Check sheet for the modelled part. Datum: model origin and axes. Units: mm. A direction names the side the tool comes from. Coordinates: 2 decimals unless noted, no trailing zeros. Loops run counter-clockwise (first coordinate to the right, second up) from the corner with the lowest first, then second, coordinate; pieces in that order, holes last. Notation, with made-up numbers: (14.25, 23) - (19.25, 23) arc R19 ccw to (19.25, 57) - close; hole circle Ø11 at (38.25, 2.5). An arc over 180 degrees is marked (long way). Write each question's results on one line, items separated by ' | '. Start each with the question number.
1. Cross-section at C-C (z = -30.5). Record the cut outline in (x, y), and give its area (3 significant figures).
2. Cross-section at A-A (x = -85). Record the cut outline in (y, z), and give its area (3 significant figures).
3. Tool access check on faces 4 (the face through (-84.931, 2.958, 18.153)), 5 (the face through (-115, 3, 1)). Record the directions out of +Z, -Z, +X, -X, +Y, -Y that give a thin tool (end or side, any length) a straight path to the whole face; none if there is none.
4. Thickness scan on line 1 (X direction, y = 2.65, z = 50); line 2 (Z direction, x = -4, y = 2.45); line 3 (Z direction, x = 40, y = 2.6). Record the ranges inside material, lowest first. Write a range as [from, to].
5. Draft check along Z on faces 1 (the face through (-108, 3, 97)), 2 (the face through (5, 3, -86)), 3 (the face through (2, 0, -1)). Enter one of: released by +Z, released by -Z, zero draft, split by the parting line, or undercut.
6. Cross-section at B-B (y = 2.75). Give the number of separate pieces and of enclosed holes in the cut face, and give its area (3 significant figures).
7. Gauge pin test, flat end, axial feed: P1, Ø3, axis at x = 61, y = 3.5, coming from the -Z side. Record the tip position at first contact, or that the pin passes through.
```python
from build123d import *

# Parameters (mm, degrees)
SKETCH1_R           = 2
SKETCH1_R_2         = 10.5
BOSS_EXTRUDE1_DEPTH = 6
SKETCH2_R           = 10
SKETCH2_R_2         = 2
CUT_EXTRUDE2_DEPTH  = 19
BOSS_EXTRUDE2_DEPTH = 6
CHAMFER1_SIZE       = 15
FILLET1_R           = 5
SKETCH4_R           = 2
CUT_EXTRUDE3_DEPTH  = 10
CUT_EXTRUDE4_DEPTH  = 10


with BuildPart() as part:
    # Sketch1 → Boss-Extrude1 (new body)
    with BuildSketch(Plane(origin=(0, 0, 0), x_dir=(1, 0, 0), z_dir=(0, 1, 0))):
        with BuildLine():
            Line((-46.904157598, -105), (46.904157598, -105))
            ThreePointArc((46.904157598, -105), (115, 0), (46.904157598, 105))
            Line((46.904157598, 105), (-46.904157598, 105))
            ThreePointArc((-46.904157598, 105), (-115, 0), (-46.904157598, -105))
        make_face()
        with Locations((-70, 80)):
            Circle(SKETCH1_R, mode=Mode.SUBTRACT)
        with Locations((70, 80)):
            Circle(SKETCH1_R, mode=Mode.SUBTRACT)
        with Locations((70, -80)):
            Circle(SKETCH1_R, mode=Mode.SUBTRACT)
        with Locations((-70, -80)):
            Circle(SKETCH1_R, mode=Mode.SUBTRACT)
        with Locations((-85, 0)):
            Circle(SKETCH1_R_2, mode=Mode.SUBTRACT)
    extrude(amount=BOSS_EXTRUDE1_DEPTH)

    # Sketch2 → Cut-Extrude2 (cut)
    with BuildSketch(Plane.XZ):
        with Locations((-50, 0)):
            Circle(SKETCH2_R)
        with Locations((-105, 0)):
            Circle(SKETCH2_R_2)
        with BuildLine():
            Line((-88.153729078, 15), (-92.680195826, 7.159929613))
            ThreePointArc((-92.680195826, 7.159929613), (-95.5, 0), (-92.680195826, -7.159929613))
            Line((-92.680195826, -7.159929613), (-88.153729078, -15))
            ThreePointArc((-88.153729078, -15), (-85, -18.153729078), (-81.846270922, -15))
            Line((-81.846270922, -15), (-77.319804174, -7.159929613))
            ThreePointArc((-77.319804174, -7.159929613), (-74.5, 0), (-77.319804174, 7.159929613))
            Line((-77.319804174, 7.159929613), (-81.846270922, 15))
            ThreePointArc((-81.846270922, 15), (-85, 18.153729078), (-88.153729078, 15))
        make_face()
        with BuildLine():
            Line((-20, -74), (30, -74))
            ThreePointArc((30, -74), (36, -80), (30, -86))
            Line((30, -86), (-20, -86))
            ThreePointArc((-20, -86), (-26, -80), (-20, -74))
        make_face()
        with BuildLine():
            Line((17.5, 74), (-17.5, 74))
            ThreePointArc((-17.5, 74), (-23.5, 80), (-17.5, 86))
            Line((-17.5, 86), (17.5, 86))
            ThreePointArc((17.5, 86), (23.5, 80), (17.5, 74))
        make_face()
    extrude(amount=-CUT_EXTRUDE2_DEPTH, mode=Mode.SUBTRACT)

    # Sketch3 → Boss-Extrude2 (add)
    with BuildSketch(Plane(origin=(0, 0, 0), x_dir=(-1, 0, 0), z_dir=(0, -1, 0))):
        with BuildLine():
            ThreePointArc((115, 0), (96.485693561, -62.574043645), (46.904157598, -105))
            Line((46.904157598, -105), (115, -105))
            Line((115, -105), (115, 0))
        make_face()
        with BuildLine():
            ThreePointArc((46.904157598, 105), (96.485693561, 62.574043645), (115, 0))
            Line((115, 0), (115, 105))
            Line((115, 105), (46.904157598, 105))
        make_face()
    extrude(amount=-BOSS_EXTRUDE2_DEPTH)

    # Chamfer1
    chamfer1_edges = [part.edges().sort_by_distance(p)[0] for p in [
        (-115, 3, 105),
        (-115, 3, -105),
    ]]
    chamfer(chamfer1_edges, length=CHAMFER1_SIZE)

    # Fillet1
    fillet1_edges = [part.edges().sort_by_distance(p)[0] for p in [
        (-115, 3, 90),
        (-115, 3, -90),
        (-100, 3, -105),
        (-100, 3, 105),
    ]]
    fillet(fillet1_edges, radius=FILLET1_R)

    # Sketch4 → Cut-Extrude3 (cut)
    with BuildSketch(Plane(origin=(0, 6, 0), x_dir=(1, 0, 0), z_dir=(0, 1, 0))):
        with Locations((-42.5, -50)):
            Circle(SKETCH4_R)
        with Locations((-97.5, -50)):
            Circle(SKETCH4_R)
        with Locations((-97.5, 50)):
            Circle(SKETCH4_R)
        with Locations((-42.5, 50)):
            Circle(SKETCH4_R)
        with Locations((-70, 70)):
            Circle(SKETCH4_R)
        with Locations((-70, -70)):
            Circle(SKETCH4_R)
        with Locations((-108, 15.259313515)):
            Circle(SKETCH4_R)
        with Locations((-108, 45.259313515)):
            Circle(SKETCH4_R)
    extrude(amount=-CUT_EXTRUDE3_DEPTH, mode=Mode.SUBTRACT)

    # Sketch5 → Cut-Extrude4 (cut)
    with BuildSketch(Plane(origin=(0, 6, 0), x_dir=(1, 0, 0), z_dir=(0, 1, 0))):
        with BuildLine():
            Line((-5, 62), (95, 62))
            ThreePointArc((95, 62), (97, 60), (95, 58))
            Line((95, 58), (-5, 58))
            ThreePointArc((-5, 58), (-7, 60), (-5, 62))
        make_face()
        with BuildLine():
            Line((-5, -62), (95, -62))
            ThreePointArc((95, -62), (97, -60), (95, -58))
            Line((95, -58), (-5, -58))
            ThreePointArc((-5, -58), (-7, -60), (-5, -62))
        make_face()
    extrude(amount=-CUT_EXTRUDE4_DEPTH, mode=Mode.SUBTRACT)


solid = part.part
```
Established:
1) outline: (-115, 0) - (110.88, 0) - (110.88, 6) - (-115, 6) - close | area: 1,360 mm^2
2) outline: (0, -105) - (6, -105) - (6, -18.15) - (0, -18.15) - close; (0, 18.15) - (6, 18.15) - (6, 105) - (0, 105) - close | area: 1,040 mm^2
3) face 4: +Y, -Y | face 5: +Z, -Z, -X, +Y, -Y
4) line 1: [-115, -99.5], [-95.5, -44.5], [-40.5, 103.56] | line 2: [-105, -86], [-74, -62], [-58, 58], [62, 74], [86, 105] | line 3: [-105, -62], [-58, 58], [62, 105]
5) face 1: released by +Z | face 2: undercut | face 3: zero draft
6) separate pieces: 1 | enclosed holes: 19 | area: 41,000 mm^2
7) P1: z = -98.41
